Input: dimensioned drawing with shaded views. Units: mm. Origin: part minimum x, y, z. A direction names the side the tool comes from. Round coordinates to 2 decimals unless told otherwise and drop trailing zeros. Loops run counter-clockwise (first coordinate to the right, second up) from the corner with the lowest first, then second, coordinate; pieces in that order, holes last. Notation, with made-up numbers: (45.5, 86.5) - (61.5, 86.5) arc R12 cw to (61.5, 95.5) - close; hole circle Ø1 at (22, 71.25). An arc over 180 degrees is marked (long way). One line per question, with ' | ' between items.
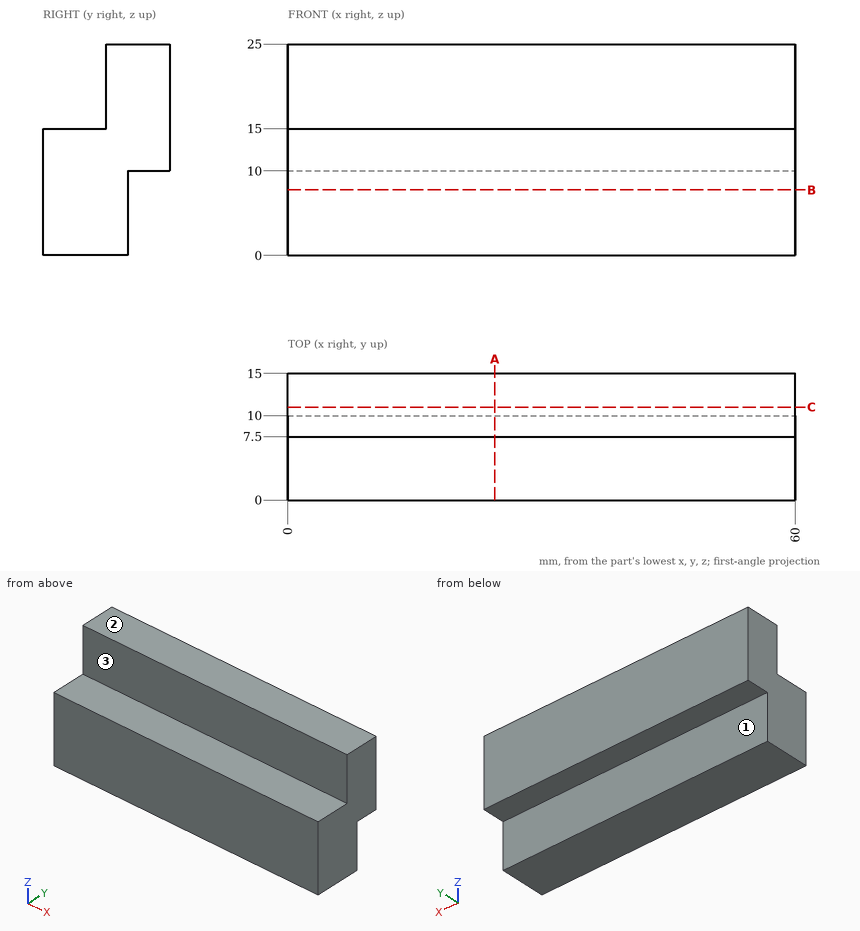
1. Section query A-A, the plane x = 24.5. Return loops of the section in (y, z), plus the area to 3 significant figures.
Worked out:
outline: (0, 0) - (10, 0) - (10, 10) - (15, 10) - (15, 25) - (7.5, 25) - (7.5, 15) - (0, 15) - close | area: 250 mm2
2. Section query B-B, the plane z = 7.75. Return loops of the section in (x, y), plus the area to 3 significant figures.
Worked out:
outline: (0, 0) - (60, 0) - (60, 10) - (0, 10) - close | area: 600 mm2
3. Section query C-C, the plane y = 11. Return loops of the section in (x, z).
Worked out:
outline: (0, 10) - (60, 10) - (60, 25) - (0, 25) - close
4. Material intervals for probe 1 along Z at (x, y) = (17, 2); probe 2 along Z at (x, y) = (57.5, 11); probe 3 along Y at (x, z) = (24, 5), sorted ascending.
Worked out:
probe 1: z = 0 to 15 | probe 2: z = 10 to 25 | probe 3: y = 0 to 10
5. Access query for the marked faces 1, 2 and 3. Directions: +Z, -Z, +X, -X, +Y, -Y. A direction counts if a zero-diameter tool reaches every point of the face in a straight line with its end or side. Return the directions, or none.
Worked out:
face 1: -Z, +X, -X, +Y | face 2: +Z, +X, -X, +Y, -Y | face 3: +Z, +X, -X, -Y
6. Contact query for flat-ended pins moving along their axis: P1, Ø1.5, axis at x = 29.5, y = 12, coming from the -Z side; P2, Ø11, axis at x = 23, z = 21, coming from the -Y side; P3, Ø3, axis at x = 28, z = 4.5, coming from the +Y side. Output: stop coordinate, or through.
Worked out:
P1: stops at z = 10 | P2: stops at y = 7.5 | P3: stops at y = 10
